```python
from build123d import *

# Parameters (mm, degrees)
SALIENTE_EXTRUIR2_DEPTH = 5
CROQUIS2_R              = 1
CORTAR_EXTRUIR1_DEPTH   = 10


with BuildPart() as part:
    # Croquis1 → Saliente-Extruir2 (new body)
    with BuildSketch(Plane.XY):
        with BuildLine():
            Line((-35, 5), (35, 5))
            ThreePointArc((35, 5), (40, 0), (35, -5))
            Line((35, -5), (-35, -5))
            ThreePointArc((-35, -5), (-40, 0), (-35, 5))
        make_face()
    extrude(amount=SALIENTE_EXTRUIR2_DEPTH)

    # Croquis2 → Cortar-Extruir1 (cut)
    with BuildSketch(Plane(origin=(0, 0, 0), x_dir=(-1, 0, 0), z_dir=(0, 0, -1))):
        Circle(CROQUIS2_R)
    extrude(amount=-CORTAR_EXTRUIR1_DEPTH, mode=Mode.SUBTRACT)


solid = part.part
```
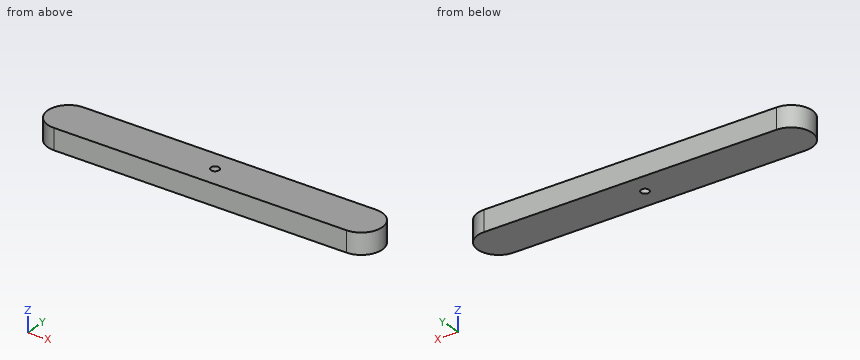
For this review, take the finished solid that the model builds, in its own axes (mm). Round coordinates to 2 decimals unless told otherwise and drop trailing zeros. Order: outer loops, then holes, each group sorted by start corner. A loop starts at its lowest first (then second) coordinate and runs counter-clockwise, first axis right, second up.
Q1. We need section D-D, the plane y = 4. Give the boundary of the cut face in (x, z), plus the area to 3 significant figures.
Findings below:
outline: (-38, 0) - (38, 0) - (38, 5) - (-38, 5) - close
area: 380 mm2
Q2. Insertion check: P1, Ø1.5, axis at y = 2.5, z = 4.5, coming from the +X side; P2, Ø1, axis at y = -3.5, z = 3, coming from the +X side; P3, Ø1, axis at y = -3.5, z = 4, coming from the -X side. Each pin has a flat end and moves straight along its axis. Give the tip position at first contact, or say it passes through.
Findings below:
P1: stops at x = 39.68
P2: stops at x = 39
P3: stops at x = -39
Q3. Wall thickness on line 1 (Y direction, x = 0, z = 1.55); line 2 (X direction, y = -4, z = 1.35); line 3 (X direction, y = 3, z = 2.4): over which ranges is each line inside the solid? List them lowest first.
Findings below:
line 1: y = -5 to -1, 1 to 5
line 2: x = -38 to 38
line 3: x = -39 to 39
Q4. We need section A-A, the plane y = 0. Give the boundary of the cut face in (x, z).
Findings below:
outline: (-40, 0) - (-1, 0) - (-1, 5) - (-40, 5) - close; (1, 0) - (40, 0) - (40, 5) - (1, 5) - close
Q5. We need section B-B, the plane x = 0. Give the boundary of the cut face in (y, z), plus the area to 3 significant figures.
Findings below:
outline: (-5, 0) - (-1, 0) - (-1, 5) - (-5, 5) - close; (1, 0) - (5, 0) - (5, 5) - (1, 5) - close
area: 40.0 mm2
Q6. We need section C-C, the plane z = 4.05. Give the boundary of the cut face in (x, y).
Findings below:
outline: (-35, -5) - (35, -5) arc R5 ccw to (35, 5) - (-35, 5) arc R5 ccw to start; hole circle Ø2 at (0, 0)
